CAD build for the part. Positions are in the model's coordinates, mm. Give positions to 0.01 mm unless a question says otherwise; leave off trailing zeros. Write each loop counter-clockwise with the first axis right and the second up, starting at its lowest first coordinate (ties: lowest second). Pieces come first, ordered by that corner, then holes. Notation, with made-up numbers: (11, 33) - (49, 33) arc R34 cw to (49, 70) - close; hole circle Ø10 at (49, 19). An arc over 180 degrees is marked (long way). Answer as a JSON object with one key per item and string values.
from build123d import *

# Parameters (mm, degrees)
SKETCH_1_W          = 165
SKETCH_1_H          = 42
SKETCH_1_R          = 7.5
SKETCH_1_R_2        = 1.65
EXTRUDE_1_DEPTH     = 3
CUT_EXTRUDE_1_DEPTH = 3
SKETCH_3_R          = 1.65
CUT_EXTRUDE_2_DEPTH = 3


with BuildPart() as part:
    # 草图1 → 凸台-拉伸1 (new body)
    with BuildSketch(Plane.XY):
        Rectangle(SKETCH_1_W, SKETCH_1_H)
        with Locations((-47, 0)):
            Circle(SKETCH_1_R, mode=Mode.SUBTRACT)
        with Locations((-75, 10)):
            Circle(SKETCH_1_R_2, mode=Mode.SUBTRACT)
        with Locations((-75, -10)):
            Circle(SKETCH_1_R_2, mode=Mode.SUBTRACT)
        with Locations((75, 10)):
            Circle(SKETCH_1_R_2, mode=Mode.SUBTRACT)
        with Locations((75, -10)):
            Circle(SKETCH_1_R_2, mode=Mode.SUBTRACT)
        with Locations((-59.374368671, 12.374368671)):
            Circle(SKETCH_1_R_2, mode=Mode.SUBTRACT)
        with Locations((-34.625631329, 12.374368671)):
            Circle(SKETCH_1_R_2, mode=Mode.SUBTRACT)
        with Locations((-34.625631329, -12.374368671)):
            Circle(SKETCH_1_R_2, mode=Mode.SUBTRACT)
        with Locations((-59.374368671, -12.374368671)):
            Circle(SKETCH_1_R_2, mode=Mode.SUBTRACT)
        with Locations(Location((59.374368671, -12.374368671, 0), (0, 0, 180))):
            Circle(SKETCH_1_R_2, mode=Mode.SUBTRACT)
        with Locations(Location((34.625631329, -12.374368671, 0), (0, 0, 180))):
            Circle(SKETCH_1_R_2, mode=Mode.SUBTRACT)
        with Locations(Location((34.625631329, 12.374368671, 0), (0, 0, 180))):
            Circle(SKETCH_1_R_2, mode=Mode.SUBTRACT)
        with Locations(Location((59.374368671, 12.374368671, 0), (0, 0, 180))):
            Circle(SKETCH_1_R_2, mode=Mode.SUBTRACT)
        with Locations(Location((47, 0, 0), (0, 0, 180))):
            Circle(SKETCH_1_R, mode=Mode.SUBTRACT)
    extrude(amount=EXTRUDE_1_DEPTH)

    # 草图2 → 切除-拉伸1 (cut)
    with BuildSketch(Plane.XY.offset(3)):
        with BuildLine():
            Line((-47, 21), (-82.5, 21))
            Line((-82.5, 21), (-82.5, -21))
            Line((-82.5, -21), (-47, -21))
            ThreePointArc((-47, -21), (-68, 0), (-47, 21))
        make_face()
        with BuildLine():
            Line((47, -21), (82.5, -21))
            Line((82.5, -21), (82.5, 21))
            Line((82.5, 21), (47, 21))
            ThreePointArc((47, 21), (68, 0), (47, -21))
        make_face()
    extrude(amount=-CUT_EXTRUDE_1_DEPTH, mode=Mode.SUBTRACT)

    # 草图3 → 切除-拉伸2 (cut)
    with BuildSketch(Plane.XY.offset(3)):
        with Locations((-26.625631329, 12.374368671)):
            Circle(SKETCH_3_R)
        with Locations((-26.625631329, -12.374368671)):
            Circle(SKETCH_3_R)
        with Locations((26.625631329, 12.374368671)):
            Circle(SKETCH_3_R)
        with Locations((26.625631329, -12.374368671)):
            Circle(SKETCH_3_R)
    extrude(amount=-CUT_EXTRUDE_2_DEPTH, mode=Mode.SUBTRACT)


solid = part.part
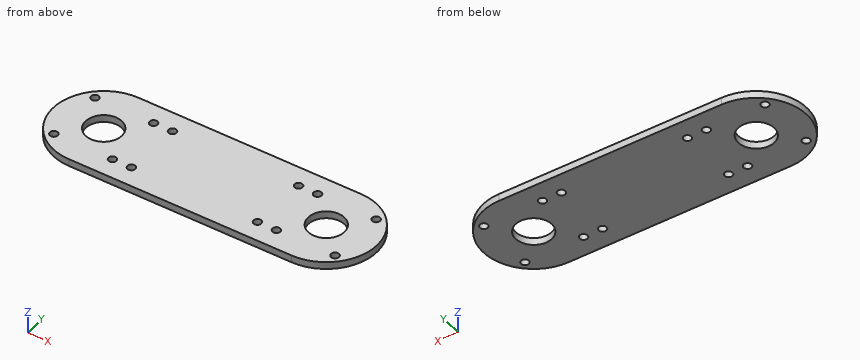
Item 1: Flat gauge pin, fed straight in: P1, Ø3, axis at x = -26.63, y = 12.37, coming from the +Z side (1 decimal). Where does the tip first touch, or does it go through?
Entries:
{"P1": "through"}
Item 2: Cut at C-C (y = -9). Give the cut face in (x, z), and give its area (3 significant figures).
Entries:
{"outline": "(-65.97, 0) - (65.97, 0) - (65.97, 3) - (-65.97, 3) - close", "area": "396 mm2"}
Item 3: Cut at A-A (y = 0). Give the cut face in (x, z), and give its area (3 significant figures).
Entries:
{"outline": "(-68, 0) - (-54.5, 0) - (-54.5, 3) - (-68, 3) - close; (-39.5, 0) - (39.5, 0) - (39.5, 3) - (-39.5, 3) - close; (54.5, 0) - (68, 0) - (68, 3) - (54.5, 3) - close", "area": "318 mm2"}
Item 4: Probe line 1 (X direction, y = -2, z = 2.05); line 2 (Y direction, x = -47, z = 0.65); line 3 (Y direction, x = 25.5, z = 1.95). List the from-to ranges inside material, lowest first. Write a range as from..to.
Entries:
{"line 1": "-67.9..-54.23, -39.77..39.77, 54.23..67.9", "line 2": "-21..-7.5, 7.5..21", "line 3": "-21..-13.58, -11.17..11.17, 13.58..21"}
Item 5: Cut at B-B (z = 1.9). State how many separate pieces and enclosed holes the cut face has, and give its area (3 significant figures).
Entries:
{"separate pieces": "1", "enclosed holes": "14", "area": "4,880 mm2"}
